Geometry check sheet. Reference: the model listing, model coordinates, mm. Face numbers are marked on the shaded views. A direction names the side the tool comes from. Give positions to 0.01 mm unless a question says otherwise; leave off trailing zeros. Loops run counter-clockwise (first coordinate to the right, second up) from the corner with the lowest first, then second, coordinate; pieces in that order, holes last.
1. Release check for a two-part mould opening along Z. For the marked faces 1, 2 and 3 record: +Z half, -Z half, draft (parallel to the pull), parting line (faces both ways), or undercut.
2. Material ranges on L1, parallel to X at y = 8.25, z = 6.5; L2, parallel to X at y = 9.5, z = 7; L3, parallel to X at y = 8.5, z = 2, recorded low to high.
3. Cross-section at A-A, the plane y = 9.5. Record the cut outline in (x, z).
4. Cross-section at B-B, the plane y = 4. Record the cut outline in (x, z).
5. Tool access check on the marked faces 4, 5 and 6. Record the directions out of +Z, -Z, +X, -X, +Y, -Y that give a thin tool (end or side, any length) a straight path to the whole face; none if there is none.
6. Go/stop test with flat-tipped pins: pin 1 Ø1.5 at (x, y) = (5, 2) entering from -Z; pin 2 Ø1 at (x, y) = (-4, 2) entering from +Z; pin 3 Ø1.5 at (y, z) = (8.5, 8.5) entering from -X. Record where each tip stops, or that it passes through.
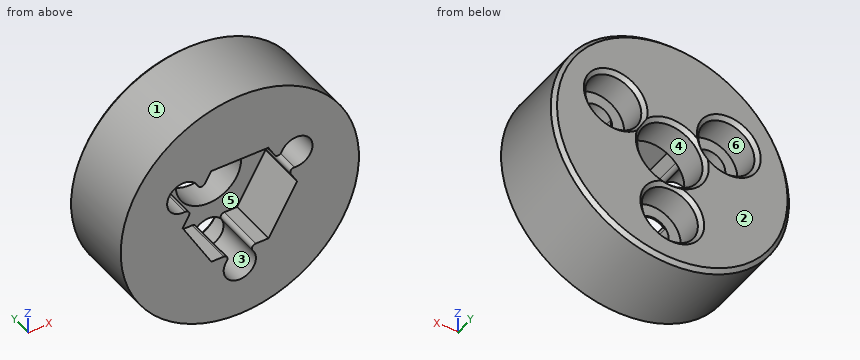
from build123d import *

# Parameters (mm, degrees)
SKETCH1_R           = 15.5
BOSS_EXTRUDE1_DEPTH = 10.6
SKETCH2_R           = 2.1
CUT_EXTRUDE1_DEPTH  = 25.348716599
SKETCH3_R           = 4.25
CUT_EXTRUDE2_DEPTH  = 25.348716599
CUT_EXTRUDE3_DEPTH  = 6.4
SKETCH5_R           = 3.65
CUT_EXTRUDE4_DEPTH  = 4
CHAMFER1_SIZE       = 0.5
FILLET_1_R          = 0.5


with BuildPart() as part:
    # Sketch1 → Boss-Extrude1 (new body)
    with BuildSketch(Plane(origin=(0, 0, 0), x_dir=(1, 0, 0), z_dir=(0, 1, 0))):
        with Locations(Location((0, 0, 0), (0, 0, 270))):
            Circle(SKETCH1_R)
    extrude(amount=BOSS_EXTRUDE1_DEPTH)

    # Sketch2 → Cut-Extrude1 (cut, through all)
    with BuildSketch(Plane(origin=(0, 10.6, 0), x_dir=(1, 0, 0), z_dir=(0, 1, 0))):
        with Locations(Location((0, 8.5, 0), (0, 0, 270))):
            Circle(SKETCH2_R)
        with Locations(Location((7.361215932, -4.25, 0), (0, 0, 270))):
            Circle(SKETCH2_R)
        with Locations(Location((-7.361215932, -4.25, 0), (0, 0, 270))):
            Circle(SKETCH2_R)
    extrude(amount=-CUT_EXTRUDE1_DEPTH, mode=Mode.SUBTRACT)

    # Sketch3 → Cut-Extrude2 (cut, through all)
    with BuildSketch(Plane(origin=(0, 10.6, 0), x_dir=(1, 0, 0), z_dir=(0, 1, 0))):
        with Locations(Location((0, 0, 0), (0, 0, 270))):
            Circle(SKETCH3_R)
    extrude(amount=-CUT_EXTRUDE2_DEPTH, mode=Mode.SUBTRACT)

    # Sketch4 → Cut-Extrude3 (cut)
    with BuildSketch(Plane.XZ):
        Polygon((3.740942098, -6.44013604), (7.447792464, 0.019682871), (3.706850366, 6.459818911), (-3.740942098, 6.44013604), (-7.447792464, -0.019682871), (-3.706850366, -6.459818911), align=None)
    extrude(amount=-CUT_EXTRUDE3_DEPTH, mode=Mode.SUBTRACT)

    # Sketch5 → Cut-Extrude4 (cut)
    with BuildSketch(Plane(origin=(0, 10.6, 0), x_dir=(1, 0, 0), z_dir=(0, 1, 0))):
        with Locations(Location((0, 8.5, 0), (0, 0, 270))):
            Circle(SKETCH5_R)
        with Locations(Location((7.361215932, -4.25, 0), (0, 0, 270))):
            Circle(SKETCH5_R)
        with Locations(Location((-7.361215932, -4.25, 0), (0, 0, 270))):
            Circle(SKETCH5_R)
    extrude(amount=-CUT_EXTRUDE4_DEPTH, mode=Mode.SUBTRACT)

    # Chamfer1
    # the kernel refuses this chamfer: 0.5 mm, written as the material it takes off along each edge
    with BuildSketch(Plane(origin=(0, 10.6, 0), x_dir=(0, 0, 1), z_dir=(-1, 0, 0))) as chamfer1_piece_1:
        Polygon((4.25 + CHAMFER1_SIZE, 0), (4.25, -CHAMFER1_SIZE), (4.25, 0), align=None)
    revolve(axis=Axis((0, 10.6, 0), (0, 1, 0)), mode=Mode.SUBTRACT)
    with BuildSketch(Plane(origin=(0, 10.6, 0), x_dir=(0, 0, 1), z_dir=(-1, 0, 0))) as chamfer1_piece_2:
        Polygon((15.5, -CHAMFER1_SIZE), (15.5 - CHAMFER1_SIZE, 0), (15.5, 0), align=None)
    revolve(axis=Axis((0, 10.6, 0), (0, 1, 0)), mode=Mode.SUBTRACT)
    with BuildSketch(Plane(origin=(0, 10.6, -8.5), x_dir=(0, 0, 1), z_dir=(-1, 0, 0))) as chamfer1_piece_3:
        Polygon((3.65 + CHAMFER1_SIZE, 0), (3.65, -CHAMFER1_SIZE), (3.65, 0), align=None)
    revolve(axis=Axis((0, 10.6, -8.5), (0, 1, 0)), mode=Mode.SUBTRACT)
    with BuildSketch(Plane(origin=(7.361215932, 10.6, 4.25), x_dir=(0, 0, 1), z_dir=(-1, 0, 0))) as chamfer1_piece_4:
        Polygon((3.65 + CHAMFER1_SIZE, 0), (3.65, -CHAMFER1_SIZE), (3.65, 0), align=None)
    revolve(axis=Axis((7.361215932, 10.6, 4.25), (0, 1, 0)), mode=Mode.SUBTRACT)
    with BuildSketch(Plane(origin=(-7.361215932, 10.6, 4.25), x_dir=(0, 0, 1), z_dir=(-1, 0, 0))) as chamfer1_piece_5:
        Polygon((3.65 + CHAMFER1_SIZE, 0), (3.65, -CHAMFER1_SIZE), (3.65, 0), align=None)
    revolve(axis=Axis((-7.361215932, 10.6, 4.25), (0, 1, 0)), mode=Mode.SUBTRACT)

    # Скругление1
    fillet_1_edges = [part.edges().sort_by_distance(p)[0] for p in [
        (5.359734874, 3.2, 3.614332183),
        (5.817474247, 3.2, 2.826321101),
        (-5.809970925, 3.2, 2.834500467),
        (-5.356402996, 3.2, 3.624919933),
        (0.450236051, 3.2, -6.44883265),
        (-0.461071251, 3.2, -6.451241034),
    ]]
    fillet(fillet_1_edges, radius=FILLET_1_R)


solid = part.part
Result:
1. face 1: parting line
1. face 2: draft
1. face 3: undercut
2. L1: x = -14.07 to -10.24, -4.49 to 4.49, 10.24 to 14.07
2. L2: x = -13.83 to -9.76, -4.96 to 4.96, 9.76 to 13.83
2. L3: x = -15.37 to -10.24, -4.49 to -3.75, 3.75 to 4.49, 10.24 to 15.37
3. outline: circle Ø31 at (0, 0); hole circle Ø7.3 at (-7.36, 4.25); hole circle Ø8.5 at (0, 0); hole circle Ø7.3 at (0, -8.5); hole circle Ø7.3 at (7.36, 4.25)
4. outline: circle Ø31 at (0, 0); hole (-7.45, -0.02) - (-3.71, -6.46) - (-2.09, -6.46) arc R0.5 cw to (-1.69, -7.25) arc R2.1 ccw (long way) to (1.68, -7.24) arc R0.5 cw to (2.08, -6.44) - (3.74, -6.44) - (7.45, 0.02) - (6.64, 1.42) arc R0.5 cw to (7.13, 2.16) arc R2.1 ccw (long way) to (5.43, 5.08) arc R0.5 cw to (4.54, 5.03) - (3.71, 6.46) - (-3.74, 6.44) - (-4.54, 5.04) arc R0.5 cw to (-5.44, 5.09) arc R2.1 ccw (long way) to (-7.11, 2.16) arc R0.5 cw to (-6.62, 1.42) - close
5. face 4: +Y, -Y
5. face 5: -Y
5. face 6: +Y
6. pin 1: stops at z = -14.91
6. pin 2: stops at z = 15.1
6. pin 3: stops at x = -13.42
